Solid Edge part; units mm, degrees
sketch "Sketch1" plane through (0, 0, 0) normal (0, 0, 1) x (1, 0, 0)
  circle A0 centre (0, 0) radius 2
  circle A1 centre (0, 0) radius 6.5
extrude "Protrusion1" add sketch "Sketch1" along normal mid plane 5
chamfer "Chamfer_1" distance 0.25 angle 45 2 edges at (-6.5, 0, 2.5) (-6.5, 0, -2.5)
sketch "Sketch2" plane through (0, 0, 0) normal (0, -1, 0) x (1, 0, 0)
  line L0 (-3.25, 2) -> (-3.25, 2.5)
  line L1 (-5.25, 2) -> (-3.25, 2)
  line L2 (-5.25, 2) -> (-5.25, 2.5)
revolve "RevolvedCutout1" cut sketch "Sketch2" angle 360 about axis through (0, 0, 54) along (0, 0, -1) material side at (-3.3, 0, 2.25)
mirror "Mirror1" about plane through (0, 0, 0) normal (0, 0, 1) of "RevolvedCutout1"
Model file for the job. Use its own axes, mm. A direction names the side the tool comes from. Coordinates: 2 decimals unless noted, no trailing zeros. Write each loop counter-clockwise with the first axis right and the second up, starting at its lowest first coordinate (ties: lowest second). Pieces come first, ordered by that corner, then holes. Notation, with made-up numbers: (79.5, 56.5) - (132.5, 56.5) arc R22 cw to (132.5, 91.5) - close; hole circle Ø7 at (89, 87). An arc over 180 degrees is marked (long way). One line per question, with ' | ' between items. Start each with the question number.
Q1. 3-axis set-ups, long thin cutter, end or side, ignore diameter. For faces 1 (the face through (2.579, -1.978, -2.254)), 2 (the face through (2.579, 1.978, 2.254)), 3 (the face through (1, -2, 2.5)): which of +Z, -Z, +X, -X, +Y, -Y reach the whole face in a straight line?
Q2. Pull direction X, two halves, no side cores. Call faces 4 (the face through (-5.158, -3.955, 0.031)), 5 (the face through (1, -2, -2.5)), 6 (the face through (-5, 1.6, -2.3)): pulls with the +X half, pulls with the -X half, needs draft (parallel to the pull), parting line crosses it, or undercut.
Q3. Cut at A-A, the plane x = 0. List the corners of the cut face in (y, z), then the cut area to 3 significant figures.
Q4. Drill centre lines: line 1 (Y direction, x = 0, z = -2.1); line 2 (Y direction, x = 0, z = -0.1); line 3 (Z direction, x = -4, y = 1.25). Where is each one in solid material? Low to high. Write a range as [from, to].
Q5. Cut at C-C, the plane z = 1.65. List the corners of the cut face in (x, y), then the cut area to 3 significant figures.
Q6. Pin check, flat tips, straight feed: pin 1 (2 mm diameter, centred on x = -5, z = -0.5, fed in from +Y); pin 2 (1 mm diameter, centred on x = 4.5, z = 0.5, fed in from -Y). Stop position of each tip, or through.
Answer below:
1) face 1: -Z | face 2: +Z | face 3: +Z, +X, -X, +Y, -Y
2) face 4: parting line crosses it | face 5: needs draft | face 6: undercut
3) outline: (-6.5, -2.25) - (-6.25, -2.5) - (-5.25, -2.5) - (-5.25, -2) - (-3.25, -2) - (-3.25, -2.5) - (-2, -2.5) - (-2, 2.5) - (-3.25, 2.5) - (-3.25, 2) - (-5.25, 2) - (-5.25, 2.5) - (-6.25, 2.5) - (-6.5, 2.25) - close; (2, -2.5) - (3.25, -2.5) - (3.25, -2) - (5.25, -2) - (5.25, -2.5) - (6.25, -2.5) - (6.5, -2.25) - (6.5, 2.25) - (6.25, 2.5) - (5.25, 2.5) - (5.25, 2) - (3.25, 2) - (3.25, 2.5) - (2, 2.5) - close | area: 40.9 mm^2
4) line 1: [-6.5, -5.25], [-3.25, -2], [2, 3.25], [5.25, 6.5] | line 2: [-6.5, -2], [2, 6.5] | line 3: [-2, 2]
5) outline: circle Ø13 at (0, 0); hole circle Ø4 at (0, 0) | area: 120 mm^2
6) pin 1: y = 5.12 | pin 2: y = -5.12
